For this review, take the finished solid that the model builds, in its own axes (mm). A direction names the side the tool comes from. Coordinates: 2 decimals unless noted, no trailing zeros. Write each loop counter-clockwise with the first axis right and the second up, starting at its lowest first coordinate (ties: lowest second). Pieces come first, ordered by that corner, then holes. Notation, with made-up numbers: M 84,-29 L 102,-29 A13 cw 102,-17 Z; hole C 38,49 d2. An arc over 180 degrees is marked long. One line per question, with ' | ' between items.
from build123d import *

# Parameters (mm, degrees)
F0_R     = 3.5
F1_DEPTH = 3
F2_R     = 5
F3_R     = 1.27


with BuildPart() as f1:
    # F0 (on Top) → F1 (new body)
    with BuildSketch(Plane.XY):
        with BuildLine():
            Line((38.5, -57.5), (38.5, 57.5))
            Line((38.5, 57.5), (-38.5, 57.5))
            Line((-38.5, 57.5), (-38.5, -57.5))
            Line((-38.5, -57.5), (-4, -57.5))
            Line((-4, -57.5), (-4, -23.507811))
            ThreePointArc((-4, -23.507811), (0, 9), (4, -23.507811))
            Line((4, -23.507811), (4, -57.5))
            Line((4, -57.5), (38.5, -57.5))
        make_face()
        with Locations((-14, -44.5)):
            Circle(F0_R, mode=Mode.SUBTRACT)
        with Locations((14, -44.5)):
            Circle(F0_R, mode=Mode.SUBTRACT)
    extrude(amount=F1_DEPTH)

    # F2
    f2_edges = [f1.edges().sort_by_distance(p)[0] for p in [
        (-38.5, 57.5, 1.5),
        (38.5, 57.5, 1.5),
        (-38.5, -57.5, 1.5),
        (38.5, -57.5, 1.5),
        (4, -57.5, 1.5),
        (-4, -57.5, 1.5),
    ]]
    fillet(f2_edges, radius=F2_R)

    # F3
    f3_edges = [f1.edges().sort_by_distance(p)[0] for p in [
        (4, -23.507811, 1.5),
        (-4, -23.507811, 1.5),
    ]]
    fillet(f3_edges, radius=F3_R)


solid = f1.part
1. Take a section at A-A on y = -38. State the section outline as (x, z) points.
Computed values:
outline: M -38.5,0 L -4,0 L -4,3 L -38.5,3 Z; M 4,0 L 38.5,0 L 38.5,3 L 4,3 Z
2. Draft analysis for pull direction X (two halves, no side actions). For faces 3 (the cylindrical face through (-37, 56.07, 1.52)), 4 (the cylindrical face through (37.07, 56, 1.52)), 5 (the cylindrical face through (-5.5, -56.07, 1.52)), state which applies: pulls with the +X half, pulls with the -X half, needs draft (parallel to the pull), parting line crosses it, or undercut.
Computed values:
face 3: pulls with the -X half | face 4: pulls with the +X half | face 5: undercut
3. For line 1 along X through (y, z) = (-28, 0.5); line 2 along X through (y, z) = (-7.5, 1.75); line 3 along Y through (x, z) = (-15, 2.4), list the stretches that pass through material, from the lowest coordinate up.
Computed values:
line 1: x = -38.5 to -4, 4 to 38.5 | line 2: x = -38.5 to -16.5, 16.5 to 38.5 | line 3: y = -57.5 to -47.85, -41.15 to -14.37, -0.63 to 57.5
4. Take a section at B-B on x = 14. State the section outline as (y, z) points.
Computed values:
outline: M -57.5,0 L -48,0 L -48,3 L -57.5,3 Z; M -41,0 L -16.23,0 L -16.23,3 L -41,3 Z; M 1.23,0 L 57.5,0 L 57.5,3 L 1.23,3 Z
5. Take a section at C-C on z = 0.85. State the section outline as (x, y) points, plus the area to 3 significant figures.
Computed values:
outline: M -38.5,-52.5 A5 ccw -33.5,-57.5 L -9,-57.5 A5 ccw -4,-52.5 L -4,-24.47 A1.27 ccw -4.89,-23.26 A16.5 cw long 4.89,-23.26 A1.27 ccw 4,-24.47 L 4,-52.5 A5 ccw 9,-57.5 L 33.5,-57.5 A5 ccw 38.5,-52.5 L 38.5,52.5 A5 ccw 33.5,57.5 L -33.5,57.5 A5 ccw -38.5,52.5 Z; hole C -14,-44.5 d7; hole C 14,-44.5 d7 | area: 7,620 mm2
6. Take a section at D-D on y = -7.5. State the section outline as (x, z) points.
Computed values:
outline: M -38.5,0 L -16.5,0 L -16.5,3 L -38.5,3 Z; M 16.5,0 L 38.5,0 L 38.5,3 L 16.5,3 Z
7. Machinability: for faces 1 (the cylindrical face through (5.5, -56.07, 1.52)), 2 (the flat face through (38.5, -1, 1)), which of the approach directions +Z, -Z, +X, -X, +Y, -Y give a long, thin tool a straight path to every point of the face, cutting with its end or side? Answer none if there is none.
Computed values:
face 1: +Z, -Z, -Y | face 2: +Z, -Z, +X, +Y, -Y
